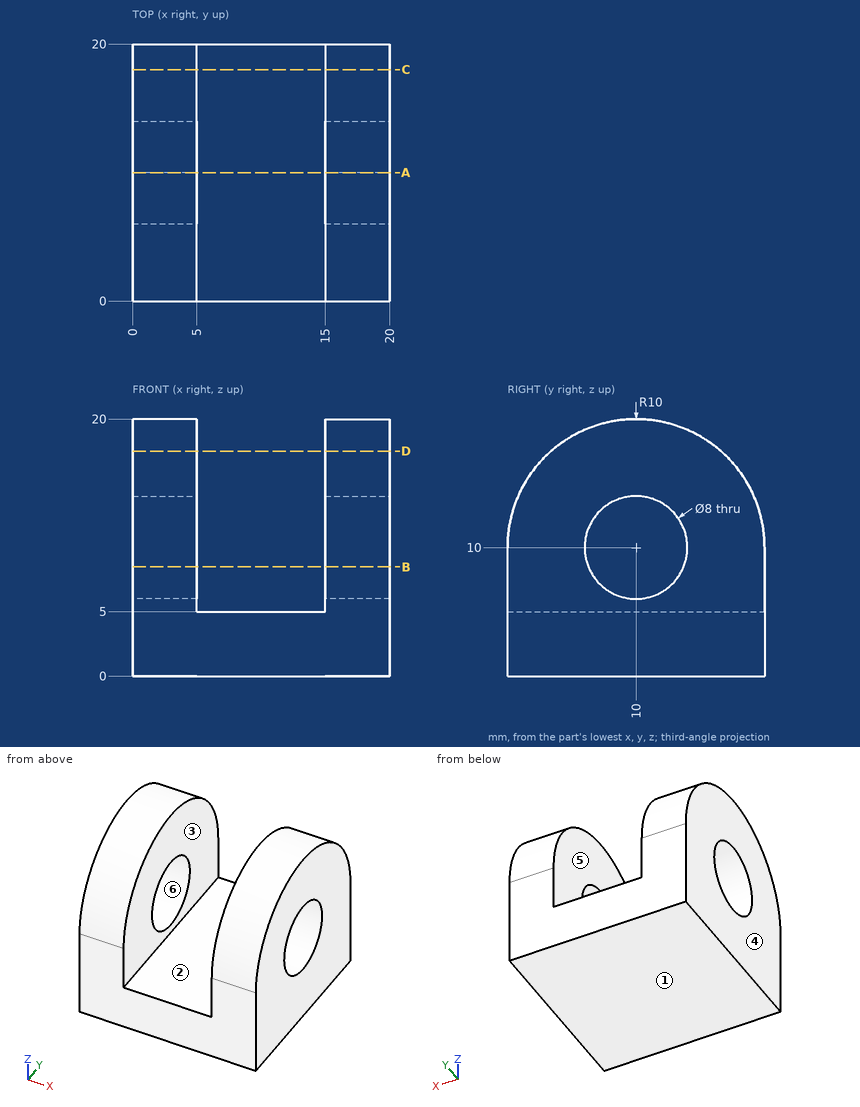
Verification items for this drawing (mm, ordinates from the low corner). A direction names the side the tool comes from. Give positions to 0.01 mm unless a question says otherwise; leave off trailing zeros. Loops run counter-clockwise (first coordinate to the right, second up) from the corner with the lowest first, then second, coordinate; pieces in that order, holes last.
1. Tool access check on the marked faces 1 and 2. Record the directions out of +Z, -Z, +X, -X, +Y, -Y that give a thin tool (end or side, any length) a straight path to the whole face; none if there is none.
Derived:
face 1: -Z, +X, -X, +Y, -Y
face 2: +Z, +Y, -Y
2. Cross-section at A-A on y = 10. Record the cut outline in (x, z).
Derived:
outline: (0, 0) - (20, 0) - (20, 6) - (15, 6) - (15, 5) - (5, 5) - (5, 6) - (0, 6) - close; (0, 14) - (5, 14) - (5, 20) - (0, 20) - close; (15, 14) - (20, 14) - (20, 20) - (15, 20) - close
3. Cross-section at D-D on z = 17.5. Record the cut outline in (x, y), and give its area (3 significant figures).
Derived:
outline: (0, 3.39) - (5, 3.39) - (5, 16.61) - (0, 16.61) - close; (15, 3.39) - (20, 3.39) - (20, 16.61) - (15, 16.61) - close
area: 132 mm2
4. Release check for a two-part mould opening along X. For the marked faces 3, 4, 5 and 6 record: +X half, -X half, draft (parallel to the pull), parting line (faces both ways), or undercut.
Derived:
face 3: undercut
face 4: -X half
face 5: undercut
face 6: draft
5. Material ranges on probe 1 along X at (y, z) = (15.75, 12); probe 2 along Y at (x, z) = (2.85, 10); probe 3 along Z at (x, y) = (10.5, 4), recorded low to high.
Derived:
probe 1: x = 0 to 5, 15 to 20
probe 2: y = 0 to 6, 14 to 20
probe 3: z = 0 to 5
6. Cross-section at C-C on y = 18. Record the cut outline in (x, z).
Derived:
outline: (0, 0) - (20, 0) - (20, 16) - (15, 16) - (15, 5) - (5, 5) - (5, 16) - (0, 16) - close
7. Cross-section at B-B on z = 8.5. Record the cut outline in (x, y).
Derived:
outline: (0, 0) - (5, 0) - (5, 6.29) - (0, 6.29) - close; (0, 13.71) - (5, 13.71) - (5, 20) - (0, 20) - close; (15, 0) - (20, 0) - (20, 6.29) - (15, 6.29) - close; (15, 13.71) - (20, 13.71) - (20, 20) - (15, 20) - close
